The figure shows three views and two pictorial views of one solid part (mm, origin at its lowest corner). Answer the questions. A direction names the side the tool comes from. Coordinates: 2 decimals unless noted, no trailing zeros. Write each loop counter-clockwise with the first axis right and the second up, starting at its lowest first coordinate (ties: lowest second). Pieces come first, ordered by that corner, then holes.
Item 1: A tool of negligible diameter and unlimited length cuts with its end or side. For the marked faces 1, 2, 3 and 4, from which of +Z, -Z, +X, -X, +Y, -Y can it reach the whole face along a straight path? Write none if from no direction.
Item 2: Section C-C (x = 15.5) is taken. Give the vertices of the cut face in (y, z) (3 decimals), then the cut area to 3 significant figures.
Item 3: Section A-A (z = 29.5) is taken. Give the vertices of the cut face in (x, y) (3 decimals), then the cut area to 3 significant figures.
Item 4: Section D-D (z = 14) is taken. Give the vertices of the cut face in (x, y) (3 decimals), then the cut area to 3 significant figures.
Item 5: Section B-B (x = 22) is taken. Give the vertices of the cut face in (y, z) (3 decimals), then the cut area to 3 significant figures.
Item 6: Straight lines are drawn through the part: probe 1 along X at (y, z) = (16, 30.5) (3 decimals); probe 2 along Z at (x, y) = (19, 23.5); probe 3 along X at (y, z) = (16.5, 36.5). For each, find the intervals that lie inside material, in ascending order.
Item 7: Each of these flat-tipped pins is pushed along its axis until it touches: P1, Ø5, axis at y = 29.5, z = 15, coming from the +X side; P2, Ø2, axis at x = 33.5, z = 20.5, coming from the -Y side; P3, Ø1, axis at y = 18.5, z = 29.5, coming from the +X side (3 decimals); P4, Ø21, axis at x = 28.5, y = 21, coming from the +Z side. Where does it stop, or does it pass through?
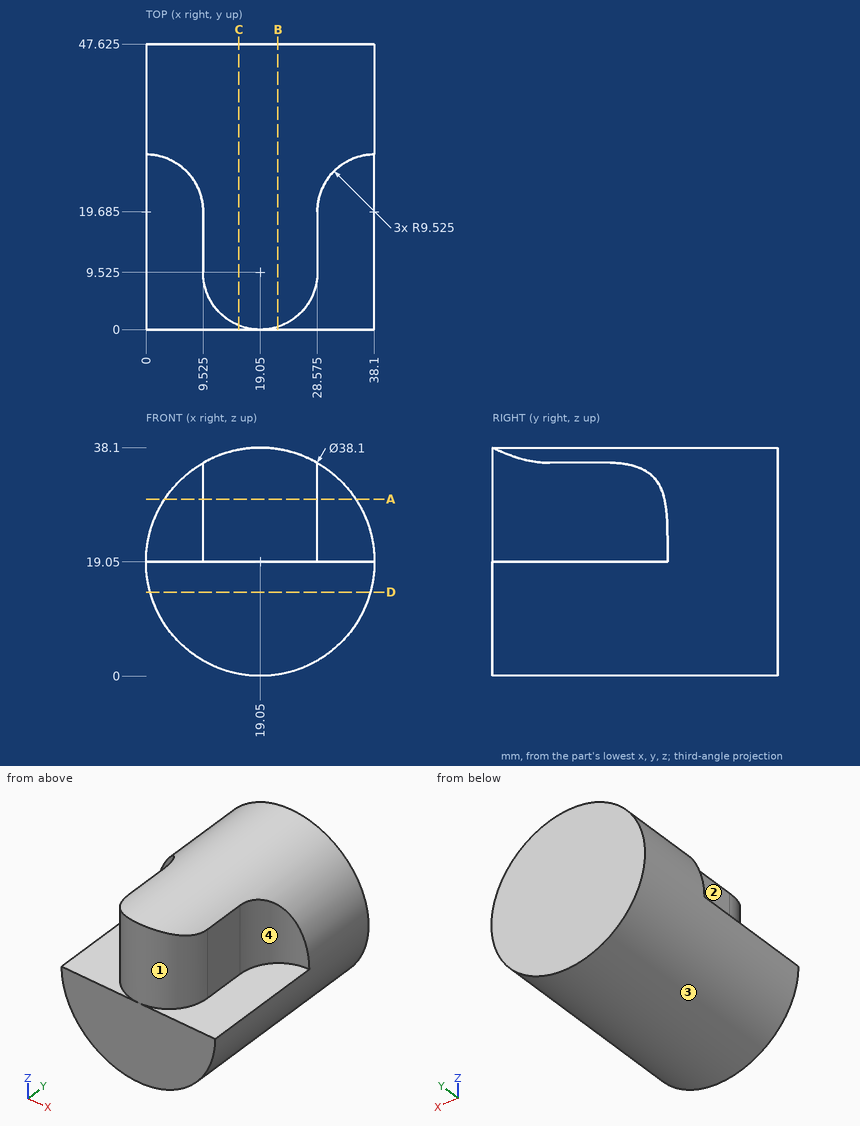
Established:
1. face 1: +Z, -Y
1. face 2: +Z, -X, -Y
1. face 3: +Y, -Y
1. face 4: +Z, +X, -Y
2. outline: (0, 0.334) - (47.625, 0.334) - (47.625, 37.766) - (0.686, 37.766) - (0.686, 19.05) - (0, 19.05) - close
2. area: 1,770 mm2
3. outline: (3.122, 28.684) arc R9.525 cw to (9.525, 19.685) - (9.525, 9.525) arc R9.525 ccw to (28.575, 9.525) - (28.575, 19.685) arc R9.525 cw to (34.978, 28.684) - (34.978, 47.625) - (3.122, 47.625) - close
3. area: 1,140 mm2
4. outline: (0.682, 0) - (37.418, 0) - (37.418, 47.625) - (0.682, 47.625) - close
4. area: 1,750 mm2
5. outline: (0, 0.23) - (47.625, 0.23) - (47.625, 37.87) - (0.468, 37.87) - (0.468, 19.05) - (0, 19.05) - close
5. area: 1,780 mm2
6. probe 1: x = 9.525 to 28.575
6. probe 2: z = 0 to 38.1
6. probe 3: x = 11.41 to 26.69
7. P1: stops at x = 38.04
7. P2: stops at y = 27.39
7. P3: stops at x = 28.575
7. P4: stops at z = 38.1
